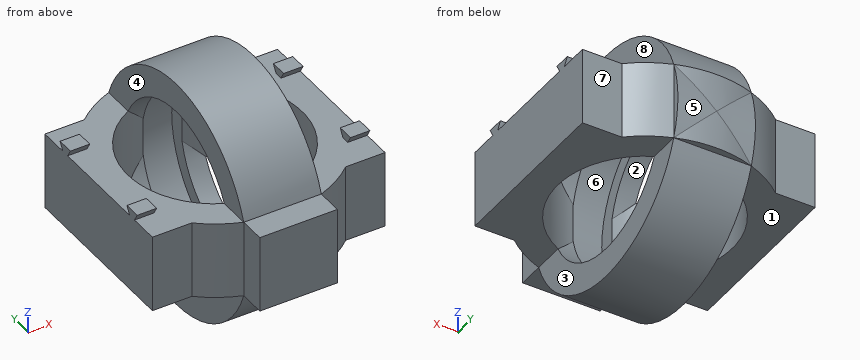
from build123d import *

# Parameters (mm, degrees)
ESQUISSE1_R                  = 60
ESQUISSE1_R_2                = 45
BOSS_EXTRU_1_DEPTH           = 40
BOSS_EXTRU_3_REACH           = 142
BOSS_EXTRU_3_END_RADIUS      = 60
ESQUISSE5_W                  = 40
ESQUISSE5_H                  = 90
BOSS_EXTRU_4_DEPTH           = 10
R_P_TITION_CIRCULAIRE1_COUNT = 2
R_P_TITION_CIRCULAIRE1_ANGLE = 90
ESQUISSE11_W                 = 20
ESQUISSE11_H                 = 15
BOSS_EXTRU_7_REACH           = 166.012
ESQUISSE17_W                 = 40
ESQUISSE17_H                 = 40


with BuildPart() as part:
    # Esquisse1 → Boss.-Extru.1 (new body)
    with BuildSketch(Plane.XY):
        Circle(ESQUISSE1_R)
        Circle(ESQUISSE1_R_2, mode=Mode.SUBTRACT)
    boss_extru_1 = extrude(amount=BOSS_EXTRU_1_DEPTH)

    # Boss.-Extru.3: up to this cylinder (the profile starts outside it)
    boss_extru_3_end = Plane(origin=(0, 0, 20), z_dir=(0, 0, -1)) * Cylinder(BOSS_EXTRU_3_END_RADIUS, 405, mode=Mode.PRIVATE)
    # Esquisse5 → Boss.-Extru.3 (add, up to the surface)
    with BuildSketch(Plane(origin=(60, 0, 0), x_dir=(0, 0, -1), z_dir=(1, 0, 0)), mode=Mode.PRIVATE) as boss_extru_3_sk1:
        with Locations((-20, 0)):
            Rectangle(ESQUISSE5_W, ESQUISSE5_H)
    boss_extru_3_tool1 = extrude(boss_extru_3_sk1.sketch, amount=-BOSS_EXTRU_3_REACH, mode=Mode.PRIVATE) - boss_extru_3_end
    boss_extru_3 = boss_extru_3_tool1.solids().sort_by_distance((60, 0, 20))[0] + boss_extru_3_tool1.solids().sort_by_distance((60, 0, 20))[1]
    add(boss_extru_3)

    # Symétrie2: Boss.-Extru.3 across plane
    add(boss_extru_3.mirror(Plane(origin=(0, 0, 0), x_dir=(0, 0, 1), z_dir=(1, 0, 0))))

    # Esquisse7 → Boss.-Extru.4 (add)
    with BuildSketch(Plane(origin=(60, 0, 0), x_dir=(0, 0, -1), z_dir=(1, 0, 0))):
        Polygon((-40, 30), (-40, 26), (-44, 23.690598923), (-44, 32.309401077), align=None)
        Polygon((-44, -32.309401077), (-40, -30), (-40, -26), (-44, -23.690598923), align=None)
    boss_extru_4 = extrude(amount=-BOSS_EXTRU_4_DEPTH)

    # Symétrie3: Boss.-Extru.4 across plane
    add(boss_extru_4.mirror(Plane(origin=(0, 0, 0), x_dir=(0, 0, 1), z_dir=(1, 0, 0))))

    # Répétition circulaire1: Boss.-Extru.1 ×2 about axis
    r_p_tition_circulaire1_axis = Axis((0, -67.301071144, 20), (0, 1, 0))
    for i in range(1, R_P_TITION_CIRCULAIRE1_COUNT):
        add(boss_extru_1.rotate(r_p_tition_circulaire1_axis, i * R_P_TITION_CIRCULAIRE1_ANGLE / (R_P_TITION_CIRCULAIRE1_COUNT - 1)))

    # Esquisse11 → Enlèvement de matière-Révolution3 (revolve, cut)
    with BuildSketch(Plane.XY.offset(20), mode=Mode.PRIVATE) as enl_vement_de_mati_re_r_volution3_sk:
        with Locations((0, -45)):
            Rectangle(ESQUISSE11_W, ESQUISSE11_H)
    revolve(enl_vement_de_mati_re_r_volution3_sk.sketch.rotate(Axis((-20, 0, 20), (1, 0, 0)), 270), axis=Axis((-20, 0, 20), (1, 0, 0)), mode=Mode.SUBTRACT)

    # Esquisse17 → Boss.-Extru.7 (add, up to next)
    with BuildSketch(Plane(origin=(0, -70, 0), x_dir=(1, 0, 0), z_dir=(0, 1, 0)), mode=Mode.PRIVATE) as boss_extru_7_sk1:
        with Locations((0, -20)):
            Rectangle(ESQUISSE17_W, ESQUISSE17_H)
    boss_extru_7_tool1 = extrude(boss_extru_7_sk1.sketch, amount=BOSS_EXTRU_7_REACH, mode=Mode.PRIVATE) - part.part
    add(boss_extru_7_tool1.solids().sort_by_distance((0, -70, 20))[0])


solid = part.part
Input: part model. Units: mm. Frame: model coordinates. Face numbers are marked on the shaded views. A direction names the side the tool comes from. Give positions to 0.01 mm unless a question says otherwise; leave off trailing zeros. Write each loop counter-clockwise with the first axis right and the second up, starting at its lowest first coordinate (ties: lowest second). Pieces come first, ordered by that corner, then holes.
Q1. Material intervals for probe 1 along Y at (x, z) = (-0.5, 20); probe 2 along X at (y, z) = (-44.5, 7); probe 3 along Z at (x, y) = (-29.5, -51), sorted ascending.
Q2. Section D-D, the plane z = -29. Output: boundary loops of the cut face in (x, y).
Q3. Pull-direction query (Y, two-part tool) for the marked faces 6, 7 and 8; classes: pulls with the +Y half, pulls with the -Y half, needs draft (parallel to the pull), parting line crosses it, or undercut.
Q4. Section C-C, the plane x = -17.5. Output: boundary loops of the cut face in (y, z).
Q5. Set-up query: the marked faces 1, 2, 3, 4 and 5. Return all of +Z, -Z, +X, -X, +Y, -Y with unobstructed straight access to the full face (end or side cutting, diameter ignored); none if empty.
Q6. Section B-B, the plane x = 28. Output: boundary loops of the cut face in (y, z).
Q7. First-contact query: P1, Ø3, axis at y = -4.5, z = 65.5, coming from the -X side; P2, Ø3, axis at x = 38, y = 30.5, coming from the +Z side; P3, Ø7, axis at x = 53, y = -29, coming from the +Z side. Flat tips, straight axial feed; report the tip coordinate or a pass-through.
Q8. Section A-A, the plane y = 0. Output: boundary loops of the cut face in (x, z).
Filled in:
1. probe 1: y = -70 to -52.5, 52.5 to 60
1. probe 2: x = -60 to -10, 10 to 60
1. probe 3: z = 0 to 40
2. outline: (-20, -34.63) - (20, -34.63) - (20, 34.63) - (-20, 34.63) - close; hole (-10, -18.85) - (10, -18.85) - (10, 18.85) - (-10, 18.85) - close
3. face 6: undercut
3. face 7: pulls with the +Y half
3. face 8: needs draft
4. outline: (-70, 0) - (-56.57, 0) arc R60 ccw to (56.57, 0) - (57.39, 0) - (57.39, 2.5) arc R60 ccw to (57.39, 37.5) - (57.39, 40) - (56.57, 40) arc R60 ccw to (-56.57, 40) - (-70, 40) - close; hole (-41.46, 2.5) arc R45 ccw to (41.46, 2.5) - (41.46, 37.5) arc R45 ccw to (-41.46, 37.5) - close
5. face 1: -Z, -X, +Y, -Y
5. face 2: none
5. face 3: -Z, +X, +Y, -Y
5. face 4: +Z, -X, +Y, -Y
5. face 5: +X, +Y
6. outline: (-53.07, 0) - (-35.23, 0) - (-35.23, 40) - (-53.07, 40) - close; (35.23, 0) - (53.07, 0) - (53.07, 40) - (35.23, 40) - close
7. P1: stops at x = -20
7. P2: stops at z = 40
7. P3: stops at z = 44
8. outline: (-60, 0) - (-45, 0) - (-45, 40) - (-60, 40) - close; (-20, -40) - (20, -40) - (20, -25) - (10, -25) - (10, -32.5) - (-10, -32.5) - (-10, -25) - (-20, -25) - close; (-20, 65) - (-10, 65) - (-10, 72.5) - (10, 72.5) - (10, 65) - (20, 65) - (20, 80) - (-20, 80) - close; (45, 0) - (60, 0) - (60, 40) - (45, 40) - close
